Study the drawing (mm; zero at the part's minimum x, y, z) and answer. A direction names the side the tool comes from. Round coordinates to 2 decimals unless told otherwise and drop trailing zeros. Loops run counter-clockwise (first coordinate to the right, second up) from the corner with the lowest first, then second, coordinate; pieces in that order, holes last. Notation, with made-up numbers: (-39.5, 39.5) -> (-22.5, 39.5) arc R5 ccw to (-22.5, 48.5) -> close; hole circle Ø1 at (49, 41.5). An arc over 180 degrees is marked (long way). Answer in a Markdown table with one row per item. Add a question column.
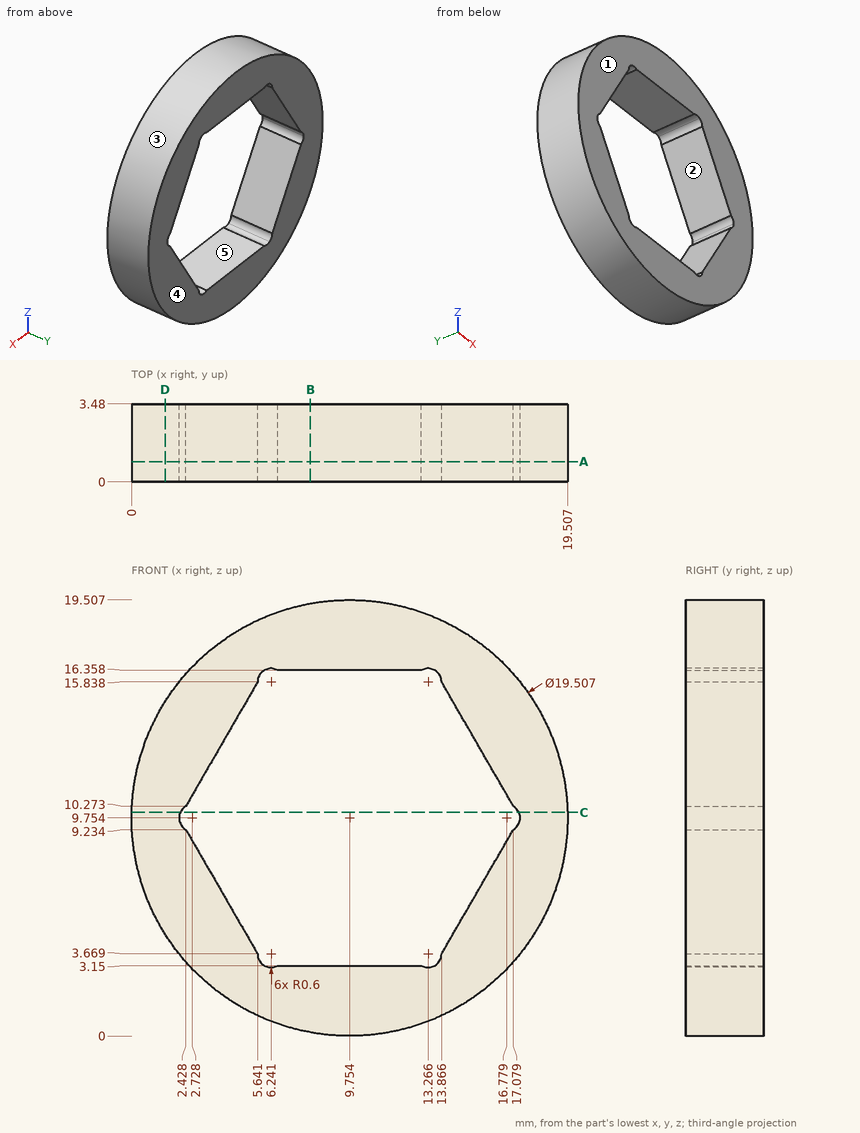
Item 1: Section C-C, the plane z = 10 is taken. Write down the section's boundary in (x, y).
Item 2: The mould has two halves that part along X. Classify the marked faces 1, 2 and 3: +X half, -X half, draft (parallel to the pull), parting line (faces both ways), or undercut.
Item 3: For the marked faces 4 and 5, determine the directions among +Z, -Z, +X, -X, +Y, -Y from which every point of the face is accessible in a straight line to the end or side of a thin tool.
Item 4: Section D-D, the plane x = 1.5 is taken. Write down the section's boundary in (y, z).
Item 5: Section A-A, the plane y = 0.9 is taken. Write down the section's boundary in (x, z), and give its area (3 significant figures).
Item 6: Flat-ended cylindrical pins translate along their axes: P1, Ø1.5, axis at x = 15, z = 9.5, coming from the +Y side; P2, Ø2, axis at x = 2, y = 3, coming from the -Z side (1 decimal); P3, Ø1, axis at y = 0.5, z = 4, coming from the +X side. Find the tip coordinate at first contact, or state that the pin passes through.
Item 7: Section B-B, the plane x = 8 is taken. Write down the section's boundary in (y, z), and give its area (3 significant figures).
Item 8: Consider L1, parallel to Z at x = 4.25, y = 1.5 (1 decimal); L2, parallel to Z at x = 15.75, y = 1.25 (1 decimal); L3, parallel to X at y = 2.1, z = 14.5 (1 decimal). Determine where each line is inside the solid, lowest interval first. Write a range as from..to.
Here are the results:
| question | item | result |
|---|---|---|
| 1 | outline | (0, 0) -> (2.18, 0) -> (2.18, 3.48) -> (0, 3.48) -> close; (17.33, 0) -> (19.5, 0) -> (19.5, 3.48) -> (17.33, 3.48) -> close |
| 2 | face 1 | draft |
| 2 | face 2 | undercut |
| 2 | face 3 | parting line |
| 3 | face 4 | +Z, -Z, +X, -X, +Y |
| 3 | face 5 | +Y, -Y |
| 4 | outline | (0, 4.56) -> (3.48, 4.56) -> (3.48, 14.95) -> (0, 14.95) -> close |
| 5 | outline | circle Ø19.51 at (9.75, 9.75); hole (2.43, 9.23) -> (5.64, 3.67) arc R0.6 ccw to (6.54, 3.15) -> (12.97, 3.15) arc R0.6 ccw to (13.87, 3.67) -> (17.08, 9.23) arc R0.6 ccw to (17.08, 10.27) -> (13.87, 15.84) arc R0.6 ccw to (12.97, 16.36) -> (6.54, 16.36) arc R0.6 ccw to (5.64, 15.84) -> (2.43, 10.27) arc R0.6 ccw to start |
| 5 | area | 147 mm² |
| 6 | P1 | passes through |
| 6 | P2 | stops at z = 2.7 |
| 6 | P3 | stops at x = 17.97 |
| 7 | outline | (0, 0.16) -> (3.48, 0.16) -> (3.48, 3.15) -> (0, 3.15) -> close; (0, 16.36) -> (3.48, 16.36) -> (3.48, 19.35) -> (0, 19.35) -> close |
| 7 | area | 20.8 mm² |
| 8 | L1 | z = 1.7..6.1, 13.4..17.8 |
| 8 | L2 | z = 2.1..6.9, 12.6..17.4 |
| 8 | L3 | x = 1.2..4.9, 14.6..18.3 |
